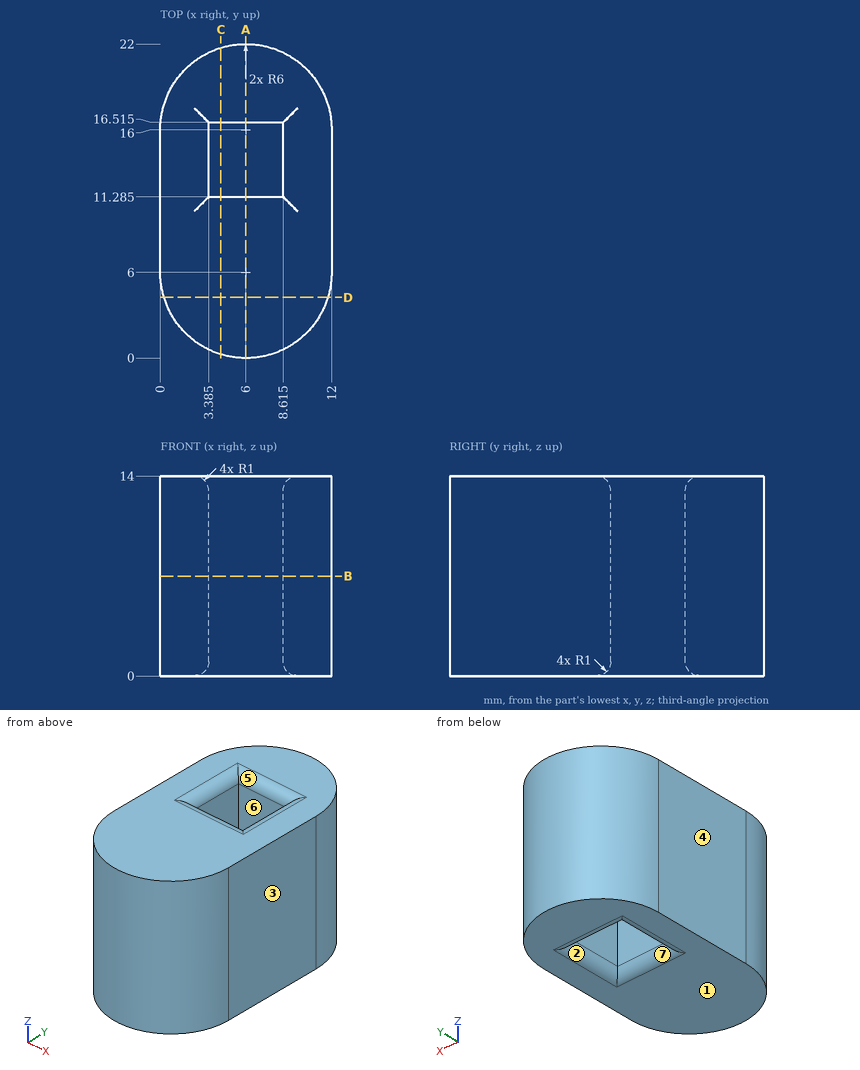
Geometry: see drawing. Coordinates: mm, zero at the bounding-box minimum. A direction names the side the tool comes from. Give positions to 0.01 mm unless a question says otherwise; leave off trailing zeros. Order: outer loops, then holes, each group sorted by start corner. A loop starts at its lowest first (then second) coordinate and runs counter-clockwise, first axis right, second up. Notation, with made-up numbers: M -40,-40 L -13,-40 A20 ccw -13,-15 Z; hole C 71,44 d9. An arc over 180 degrees is marked long. Answer as a JSON object with one key per item and string values.
1. Cut plane B-B, the plane z = 7. Output: boundary loops of the cut face in (x, y) (3 decimals), and give its area (3 significant figures).
Result sheet:
{"outline": "M 0,6 A6 ccw 12,6 L 12,16 A6 ccw 0,16 Z; hole M 3.385,11.285 L 8.615,11.285 L 8.615,16.515 L 3.385,16.515 Z", "area": "206 mm²"}
2. Ray query, line 1 (Y direction, x = 6.25, z = 11.25) (3 decimals); line 2 (X direction, y = 14.5, z = 6.5) (3 decimals); line 3 (Y direction, x = 3.5, z = 10) (3 decimals). Return the intervals inside material, ascending. Write a range as [from, to].
Result sheet:
{"line 1": "[0.005, 11.285], [16.515, 21.995]", "line 2": "[0, 3.385], [8.615, 12]", "line 3": "[0.546, 11.285], [16.515, 21.454]"}
3. First-contact query: P1, Ø1.6, axis at x = 5, z = 7.5, coming from the +Y side; P2, Ø3, axis at x = 10.5, z = 7, coming from the +Y side; P3, Ø3, axis at y = 4, z = 5.5, coming from the +X side. Flat tips, straight axial feed; report the tip coordinate or a pass-through.
Result sheet:
{"P1": "y = 22", "P2": "y = 21.2", "P3": "x = 11.98"}
4. Cut plane A-A, the plane x = 6. Output: boundary loops of the cut face in (y, z) (3 decimals).
Result sheet:
{"outline": "M 0,0 L 10.285,0 A1 ccw 11.285,1 L 11.285,13 A1 ccw 10.285,14 L 0,14 Z; M 16.515,1 A1 ccw 17.515,0 L 22,0 L 22,14 L 17.515,14 A1 ccw 16.515,13 Z"}
5. Reachability of the marked faces 5, 6 and 7 from +Z, -Z, +X, -X, +Y, -Y: full face, straight path, thin tool, end or side. Return the list, or none.
Result sheet:
{"face 5": "+Z", "face 6": "+Z, -Z", "face 7": "-Z"}
6. Cut plane D-D, the plane y = 4.25. Output: boundary loops of the cut face in (x, z).
Result sheet:
{"outline": "M 0.26,0 L 11.74,0 L 11.74,14 L 0.26,14 Z"}
7. Cut plane C-C, the plane x = 4.25. Output: boundary loops of the cut face in (y, z) (3 decimals).
Result sheet:
{"outline": "M 0.261,0 L 10.285,0 A1 ccw 11.285,1 L 11.285,13 A1 ccw 10.285,14 L 0.261,14 Z; M 16.515,1 A1 ccw 17.515,0 L 21.739,0 L 21.739,14 L 17.515,14 A1 ccw 16.515,13 Z"}
8. Pull-direction query (X, two-part tool) for the marked faces 1, 2, 3 and 4; classes: +X half, -X half, draft (parallel to the pull), parting line (faces both ways), or undercut.
Result sheet:
{"face 1": "draft", "face 2": "undercut", "face 3": "+X half", "face 4": "-X half"}
